```python
from build123d import *

# Parameters (mm, degrees)
SKETCH_1_R          = 18.38
EXTRUDE_1_DEPTH     = 22.17
SKETCH_2_R          = 16.365
EXTRUDE_2_DEPTH     = 22.22
SKETCH_3_R          = 5.98
EXTRUDE_3_DEPTH     = 5.7
SKETCH_4_R          = 3
EXTRUDE_4_DEPTH     = 14.96
SKETCH_5_W          = 1.304796907
SKETCH_5_H          = 4.648976657
CUT_EXTRUDE_1_DEPTH = 12
SKETCH_6_R          = 1.255
CUT_EXTRUDE_2_DEPTH = 3
CUT_EXTRUDE_3_DEPTH = 1
FILLET_1_R          = 0.5
FILLET_3_R          = 0.5
SKETCH_8_W          = 0.5
SKETCH_8_H          = 2.93
EXTRUDE_5_DEPTH     = 6.44
SKETCH_9_R          = 3.775
EXTRUDE_6_DEPTH     = 2.95
CUT_EXTRUDE_4_DEPTH = 2.95
SKETCH_11_W         = 1.680936825
SKETCH_11_H         = 0.866217562
CUT_EXTRUDE_5_DEPTH = 37.95
FILLET_4_R          = 0.5


with BuildPart() as part:
    # Эскиз1 → Бобышка-Вытянуть1 (new body)
    with BuildSketch(Plane.XY):
        Circle(SKETCH_1_R)
    extrude(amount=EXTRUDE_1_DEPTH)

    # Эскиз2 → Бобышка-Вытянуть2 (add)
    with BuildSketch(Plane.XY.offset(22.17)):
        Circle(SKETCH_2_R)
    extrude(amount=EXTRUDE_2_DEPTH)

    # Эскиз3 → Бобышка-Вытянуть3 (add)
    with BuildSketch(Plane(origin=(0, 0, 0), x_dir=(-1, 0, 0), z_dir=(0, 0, -1))):
        with Locations((7.9, 0)):
            Circle(SKETCH_3_R)
    extrude(amount=EXTRUDE_3_DEPTH)

    # Эскиз4 → Бобышка-Вытянуть4 (add)
    with BuildSketch(Plane(origin=(0, 0, -5.7), x_dir=(-1, 0, 0), z_dir=(0, 0, -1))):
        with Locations((7.9, 0)):
            Circle(SKETCH_4_R)
    extrude(amount=EXTRUDE_4_DEPTH)

    # Эскиз5 → Вырез-Вытянуть1 (cut)
    with BuildSketch(Plane(origin=(0, 0, -20.66), x_dir=(-1, 0, 0), z_dir=(0, 0, -1))):
        with Locations((11.042398454, -0.267988811)):
            Rectangle(SKETCH_5_W, SKETCH_5_H)
    extrude(amount=-CUT_EXTRUDE_1_DEPTH, mode=Mode.SUBTRACT)

    # Эскиз6 → Вырез-Вытянуть2 (cut)
    with BuildSketch(Plane(origin=(0, 0, 0), x_dir=(-1, 0, 0), z_dir=(0, 0, -1))):
        with Locations((0, -15.605)):
            Circle(SKETCH_6_R)
        with Locations((-13.514326426, -7.8025)):
            Circle(SKETCH_6_R)
        with Locations((-13.514326426, 7.8025)):
            Circle(SKETCH_6_R)
        with Locations((0, 15.605)):
            Circle(SKETCH_6_R)
        with Locations((13.514326426, 7.8025)):
            Circle(SKETCH_6_R)
        with Locations((13.514326426, -7.8025)):
            Circle(SKETCH_6_R)
    extrude(amount=-CUT_EXTRUDE_2_DEPTH, mode=Mode.SUBTRACT)

    # Эскиз7 → Вырез-Вытянуть3 (cut)
    with BuildSketch(Plane(origin=(0, 0, 0), x_dir=(-1, 0, 0), z_dir=(0, 0, -1))):
        with BuildLine():
            ThreePointArc((7.9, 6.731145279), (1.168854721, 0), (7.9, -6.731145279))
            ThreePointArc((7.9, -6.731145279), (-14.190210328, 0), (7.9, 6.731145279))
        make_face()
    extrude(amount=-CUT_EXTRUDE_3_DEPTH, mode=Mode.SUBTRACT)

    # Скругление1
    fillet_1_edges = [part.edges().sort_by_distance(p)[0] for p in [
        (14.190210328, 0, 1),
        (-1.168854721, 0, 1),
    ]]
    fillet(fillet_1_edges, radius=FILLET_1_R)

    # Скругление3
    fillet_3_edges = [part.edges().sort_by_distance(p)[0] for p in [
        (-1.92, 0, -5.7),
    ]]
    fillet(fillet_3_edges, radius=FILLET_3_R)

    # Эскиз8 → Бобышка-Вытянуть5 (add)
    with BuildSketch(Plane.XY.offset(44.39)):
        with Locations((-12.585, 0)):
            Rectangle(SKETCH_8_W, SKETCH_8_H)
        with Locations((12.585, 0)):
            Rectangle(SKETCH_8_W, SKETCH_8_H)
    extrude(amount=EXTRUDE_5_DEPTH)

    # Эскиз9 → Бобышка-Вытянуть6 (add)
    with BuildSketch(Plane.XY.offset(44.39)):
        Circle(SKETCH_9_R)
    extrude(amount=EXTRUDE_6_DEPTH)

    # Эскиз10 → Вырез-Вытянуть4 (cut)
    with BuildSketch(Plane.XY.offset(44.39)):
        with BuildLine():
            ThreePointArc((-4.166478649, 2.760889391), (-4.998205134, 0), (-4.166478649, -2.760889391))
            ThreePointArc((-4.166478649, -2.760889391), (-3.573206608, -2.881623675), (-3.451786459, -2.288491624))
            ThreePointArc((-3.451786459, -2.288491624), (-4.141500171, 0), (-3.451786459, 2.288491624))
            ThreePointArc((-3.451786459, 2.288491624), (-3.573206608, 2.881623675), (-4.166478649, 2.760889391))
        make_face()
        with BuildLine():
            ThreePointArc((2.760889391, 4.166478649), (0, 4.998205134), (-2.760889391, 4.166478649))
            ThreePointArc((-2.760889391, 4.166478649), (-2.881623675, 3.573206608), (-2.288491624, 3.451786459))
            ThreePointArc((-2.288491624, 3.451786459), (0, 4.141500171), (2.288491624, 3.451786459))
            ThreePointArc((2.288491624, 3.451786459), (2.881623675, 3.573206608), (2.760889391, 4.166478649))
        make_face()
        with BuildLine():
            ThreePointArc((4.166478649, -2.760889391), (4.998205134, 0), (4.166478649, 2.760889391))
            ThreePointArc((4.166478649, 2.760889391), (3.573206608, 2.881623675), (3.451786459, 2.288491624))
            ThreePointArc((3.451786459, 2.288491624), (4.141500171, 0), (3.451786459, -2.288491624))
            ThreePointArc((3.451786459, -2.288491624), (3.573206608, -2.881623675), (4.166478649, -2.760889391))
        make_face()
        with BuildLine():
            ThreePointArc((-2.760889391, -4.166478649), (0, -4.998205134), (2.760889391, -4.166478649))
            ThreePointArc((2.760889391, -4.166478649), (2.881623675, -3.573206608), (2.288491624, -3.451786459))
            ThreePointArc((2.288491624, -3.451786459), (0, -4.141500171), (-2.288491624, -3.451786459))
            ThreePointArc((-2.288491624, -3.451786459), (-2.881623675, -3.573206608), (-2.760889391, -4.166478649))
        make_face()
    extrude(amount=-CUT_EXTRUDE_4_DEPTH, mode=Mode.SUBTRACT)

    # Эскиз11 → Вырез-Вытянуть5 (cut)
    with BuildSketch(Plane.ZY.offset(12.835)):
        with Locations((49.383028143, 0)):
            Rectangle(SKETCH_11_W, SKETCH_11_H)
    extrude(amount=-CUT_EXTRUDE_5_DEPTH, mode=Mode.SUBTRACT)

    # Скругление4
    fillet_4_edges = [part.edges().sort_by_distance(p)[0] for p in [
        (-12.585, 1.465, 50.83),
        (-12.585, -1.465, 50.83),
        (12.585, 1.465, 50.83),
        (12.585, -1.465, 50.83),
    ]]
    fillet(fillet_4_edges, radius=FILLET_4_R)


solid = part.part
```
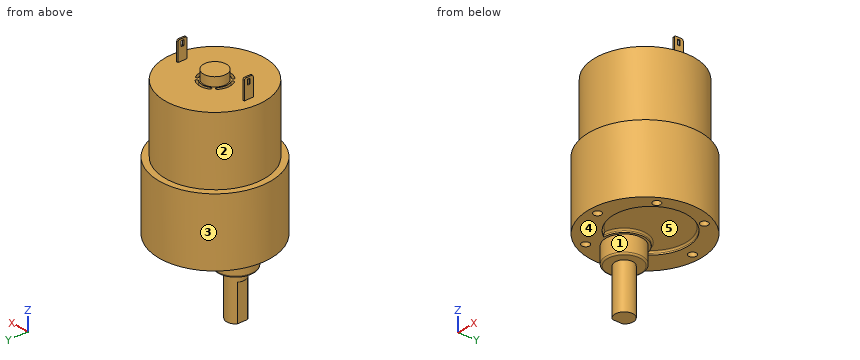
Part model, mm, in its own coordinate system. Face numbers are marked on the shaded views. A direction names the side the tool comes from. Round coordinates to 2 decimals unless told otherwise and drop trailing zeros. Loops run counter-clockwise (first coordinate to the right, second up) from the corner with the lowest first, then second, coordinate; pieces in that order, holes last.
1. 3-axis set-ups, long thin cutter, end or side, ignore diameter. For the marked faces 1 and 2: which of +Z, -Z, +X, -X, +Y, -Y reach the whole face in a straight line?
Solutions:
face 1: -Z
face 2: +Z
2. Drill centre lines: line 1 along Z through (x, y) = (-9, -6); line 2 along Z through (x, y) = (-13.5, 11.5); line 3 along Y through (x, z) = (0.5, 11). Where is each one in solid material? Low to high.
Solutions:
line 1: z = 0 to 44.39
line 2: z = 0 to 22.17
line 3: y = -18.37 to 18.37
3. Flat gauge pins, fed straight in: pin 1 (0.8 mm diameter, centred on x = -13.5, y = 8, fed in from -Z); pin 2 (1.5 mm diameter, centred on y = -0.5, z = 46.5, fed in from -X) (3 decimals); pin 3 (3 mm diameter, centred on y = -14, z = 11, fed in from +X). Where does each tip first touch, or does it go through?
Solutions:
pin 1: stops at z = 3
pin 2: stops at x = -12.835
pin 3: stops at x = 13.47
4. Two-plate mould, pull along X, no slides. Class the marked faces 3, 4 and 5: pulls with the +X half, pulls with the -X half, needs draft (parallel to the pull), parting line crosses it, or undercut.
Solutions:
face 3: parting line crosses it
face 4: needs draft
face 5: undercut
5. Slice it at B-B (z = 33). Give the cut face in (x, y) (3 decimals).
Solutions:
outline: circle Ø32.73 at (0, 0)
6. Slice it at A-A (z = 18). Give the cut face in (x, y), and give its area (3 significant figures).
Solutions:
outline: circle Ø36.76 at (0, 0)
area: 1,060 mm2
